from build123d import *

# Parameters (mm, degrees)
SKETCH1_R             = 52.3875
SKETCH1_R_2           = 23.5
BOSS_EXTRUDE1_DEPTH   = 11.43
M6_CLEARANCE_HOLE1_D  = 6.6
F_5_0MM_DOWEL_HOLE1_D = 5
CIRPATTERN1_COUNT     = 4


with BuildPart() as part:
    # Sketch1 → Boss-Extrude1 (new body)
    with BuildSketch(Plane(origin=(0, 0, 0), x_dir=(1, 0, 0), z_dir=(0, 1, 0))):
        with BuildLine():
            Line((-205.575185514, -163.900359311), (-162.418239385, -163.900359311))
            ThreePointArc((-162.418239385, -163.900359311), (-141.68491097, -175.086974107), (-118.273664056, -177.718470957))
            Line((-118.273664056, -177.718470957), (57.534589587, -163.713698748))
            ThreePointArc((57.534589587, -163.713698748), (88.232990974, -142.03141304), (83.918702981, -104.696439083))
            Line((83.918702981, -104.696439083), (17.613541845, -17.566035058))
            ThreePointArc((17.613541845, -17.566035058), (9.029109122, -13.862322556), (1.412558245, -19.284326264))
            Line((1.412558245, -19.284326264), (-12.176603989, -48.212200061))
            ThreePointArc((-12.176603989, -48.212200061), (-33.518744337, -68.231765471), (-62.780706514, -68.14502812))
            Line((-62.780706514, -68.14502812), (-207.974881785, -9.956762437))
            ThreePointArc((-207.974881785, -9.956762437), (-218.104712161, -11.917535088), (-220.5058623, -21.95210388))
            Line((-220.5058623, -21.95210388), (-186.782347933, -118.053350031))
            ThreePointArc((-186.782347933, -118.053350031), (-186.837480234, -128.184816063), (-193.296838451, -135.990348392))
            Line((-193.296838451, -135.990348392), (-210.444169906, -146.188869465))
            ThreePointArc((-210.444169906, -146.188869465), (-214.759463951, -156.900167147), (-205.575185514, -163.900359311))
        make_face()
        with Locations(Location((-123.19, -116.001477372, 0), (0, 0, 270))):
            Circle(SKETCH1_R, mode=Mode.SUBTRACT)
        with Locations(Location((54.61, -127, 0), (0, 0, 270))):
            Circle(SKETCH1_R_2, mode=Mode.SUBTRACT)
    extrude(amount=BOSS_EXTRUDE1_DEPTH)

    # M6 Clearance Hole1 (through all)
    with Locations(Plane(origin=(0, 0, 0), x_dir=(-1, 0, 0), z_dir=(0, -1, 0))):
        with Locations((-10.033704867, -23.334197365), (211.518182886, -18.798178744), (205.575185514, -154.375359311)):
            Hole(M6_CLEARANCE_HOLE1_D / 2)

    # Ø5.0mm Dowel Hole1 (through all)
    with Locations(Plane(origin=(0, 0, 0), x_dir=(-1, 0, 0), z_dir=(0, -1, 0))):
        with Locations((123.19, -173.151477372)):
            f_5_0mm_dowel_hole1 = Hole(F_5_0MM_DOWEL_HOLE1_D / 2)

    # CirPattern1: Ø5.0mm Dowel Hole1 ×4 about axis
    cirpattern1_axis = Axis((-123.19, 0, 116.001477372), (0, 1, 0))
    for i in range(1, CIRPATTERN1_COUNT):
        add(f_5_0mm_dowel_hole1.rotate(cirpattern1_axis, i * 360 / CIRPATTERN1_COUNT), mode=Mode.SUBTRACT)


solid = part.part
Part model, mm, in its own coordinate system. A direction names the side the tool comes from. Round coordinates to 2 decimals unless told otherwise and drop trailing zeros. Write each loop counter-clockwise with the first axis right and the second up, starting at its lowest first coordinate (ties: lowest second). Pieces come first, ordered by that corner, then holes. Notation, with made-up numbers: (80.25, 66) - (94.25, 66) arc R33 ccw to (94.25, 98) - close; hole circle Ø9 at (82, 60). An arc over 180 degrees is marked (long way). Use CSV: the item, a comma, the result in double quotes.
Item 1: Slice it at C-C, the plane z = 100. Write the cut outline in (x, y), then the cut area to 3 significant figures.
Results list:
outline,"(-193.12, 0) - (-173.07, 0) - (-173.07, 11.43) - (-193.12, 11.43) - close; (-73.31, 0) - (80.34, 0) - (80.34, 11.43) - (-73.31, 11.43) - close"
area,"1,990 mm²"
Item 2: Slice it at A-A, the plane x = 50. Write the cut outline in (y, z), then the cut area to 3 significant figures.
Results list:
outline,"(0, 60.12) - (11.43, 60.12) - (11.43, 103.96) - (0, 103.96) - close; (0, 150.04) - (11.43, 150.04) - (11.43, 164.31) - (0, 164.31) - close"
area,"664 mm²"
Item 3: Slice it at B-B, the plane z = 127. Write the cut outline in (x, y).
Results list:
outline,"(-186.46, 0) - (-174.41, 0) - (-174.41, 11.43) - (-186.46, 11.43) - close; (-71.97, 0) - (31.11, 0) - (31.11, 11.43) - (-71.97, 11.43) - close; (78.11, 0) - (91.44, 0) - (91.44, 11.43) - (78.11, 11.43) - close"
Item 4: Wall check: L1, parallel to X at y = 4, z = 125; L2, parallel to X at y = 9.5, z = 57.5; L3, parallel to X at y = 10.5, z = 63.5. Give the ranges that are in metal, low to high.
Results list:
L1,"x = -186.06 to -174.8, -71.58 to 31.2, 78.02 to 91.39"
L2,"x = -208.03 to -125.29, -121.09 to -89.34, -18.26 to 48"
L3,"x = -205.93 to -74.37, -24.86 to 52.57"
Item 5: Flat gauge pins, fed straight in: P1, Ø5.5, axis at x = 10.03, z = 23.33, coming from the -Y side; P2, Ø8.5, axis at x = -205.58, z = 154.38, coming from the -Y side; P3, Ø3, axis at x = 6.5, y = 9, coming from the +Z side; P4, Ø1.5, axis at x = 9, y = 5.5, coming from the +Z side. Where does each tip first touch, or does it go through?
Results list:
P1,"passes through"
P2,"stops at y = 0"
P3,"stops at z = 167.9"
P4,"stops at z = 167.64"
Item 6: Pull direction Z, two halves, no side cores. Call faces 4 (the flat face through (-134.36, 5.63, 39.46)), 5 (the flat face through (-203.88, 5.63, 69.33)), 6 (the flat face through (-31.6, 5.635, 170.814)): pulls with the +Z half, pulls with the -Z half, needs draft (parallel to the pull), parting line crosses it, or undercut.
Results list:
face 4,"pulls with the -Z half"
face 5,"undercut"
face 6,"pulls with the +Z half"
Item 7: Slice it at D-D, the plane y = 4. Count the separate pieces of the cut face and the enclosed holes in it, then the cut area to 3 significant figures.
Results list:
separate pieces,"1"
enclosed holes,"9"
area,"24,700 mm²"
Item 8: Tool access for faces 1 (the flat face through (-201.75, 5.63, 141.02)), 2 (the flat face through (-184, 6, 163.9)), 3 (the flat face through (-5.29, 5.63, 33.55)): list every direction of +Z, -Z, +X, -X, +Y, -Y with a clear straight run to the whole face (end or side of a thin tool).
Results list:
face 1,"-X, +Y, -Y"
face 2,"+Z, -X, +Y, -Y"
face 3,"-Z, +Y, -Y"
